Build history of the part. All positions in model axes, mm. A direction names the side the tool comes from. Round coordinates to 2 decimals unless told otherwise and drop trailing zeros. Loops run counter-clockwise (first coordinate to the right, second up) from the corner with the lowest first, then second, coordinate; pieces in that order, holes last. Notation, with made-up numbers: (-27.75, 80) - (7.25, 80) arc R29 cw to (7.25, 119) - close; hole circle Ø9 at (54, 23.25). An arc over 180 degrees is marked (long way). Answer as CSV lines item,"result". Start each with the question number.
```python
from build123d import *

# Parameters (mm, degrees)
F0_W           = 203.2
F0_H           = 76.2
F1_DEPTH       = 50.8
F3_D           = 13.4874
F3_CBORE_D     = 22.225
F3_CBORE_DEPTH = 38.1


with BuildPart() as f1:
    # F0 (on Top) → F1 (new body)
    with BuildSketch(Plane.XY):
        Rectangle(F0_W, F0_H)
    extrude(amount=F1_DEPTH)

    # F3 (through all)
    with Locations(Plane.XY.offset(50.8)):
        with Locations((-49.2125, -14.224), (49.2125, -14.224)):
            CounterBoreHole(F3_D / 2, F3_CBORE_D / 2, F3_CBORE_DEPTH)


solid = f1.part
```
Q1. Wall check: probe 1 along X at (y, z) = (-5, 39); probe 2 along Z at (x, y) = (-40, -10.5); probe 3 along X at (y, z) = (-9.5, 19). Give the ranges that are in metal, low to high. Write a range as [from, to].
Q2. Two-plate mould, pull along X, no slides. Class faces 1 (the cylindrical face through (42.983, -16.807, 6.261)), 2 (the flat face through (-1, 38.1, 25)), 3 (the flat face through (101.6, -1, 25)): released by +X, released by -X, zero draft, split by the parting line, or undercut.
Q3. Band-saw the part on B-B, the plane y = -10. List the corners of the cut face in (x, z), then the cut area to 3 significant figures.
Q4. Tool access for faces 4 (the flat face through (-101.6, -1, 25)), 5 (the cylindrical face through (-50.659, -3.206, 32.017)): list every direction of +Z, -Z, +X, -X, +Y, -Y with a clear straight run to the whole face (end or side of a thin tool).
Q5. Band-saw the part on C-C, the plane z = 39. List the corners of the cut face in (x, y) (1 decimal).
Q6. Band-saw the part on A-A, the plane x = -48. List the corners of the cut face in (y, z).
Q7. Pin check, flat tip, straight feed: pin 1 Ø6.5 at (x, y) = (-53.5, -10.5) entering from +Z. Stop position of the tip, or through.
Reported:
1,probe 1,"x = [-101.6, -55.41], [-43.02, 43.02], [55.41, 101.6]"
1,probe 2,"z = [0, 12.7]"
1,probe 3,"x = [-101.6, -59.27], [-39.15, 39.15], [59.27, 101.6]"
2,face 1,"undercut"
2,face 2,"zero draft"
2,face 3,"released by +X"
3,outline,"(-101.6, 0) - (-54.47, 0) - (-54.47, 12.7) - (-59.49, 12.7) - (-59.49, 50.8) - (-101.6, 50.8) - close; (-43.96, 0) - (43.96, 0) - (43.96, 12.7) - (38.93, 12.7) - (38.93, 50.8) - (-38.93, 50.8) - (-38.93, 12.7) - (-43.96, 12.7) - close; (54.47, 0) - (101.6, 0) - (101.6, 50.8) - (59.49, 50.8) - (59.49, 12.7) - (54.47, 12.7) - close"
3,area,"8,490 mm2"
4,face 4,"+Z, -Z, -X, +Y, -Y"
4,face 5,"+Z"
5,outline,"(-101.6, -38.1) - (101.6, -38.1) - (101.6, 38.1) - (-101.6, 38.1) - close; hole circle Ø22.2 at (-49.2, -14.2); hole circle Ø22.2 at (49.2, -14.2)"
6,outline,"(-38.1, 0) - (-20.86, 0) - (-20.86, 12.7) - (-25.27, 12.7) - (-25.27, 50.8) - (-38.1, 50.8) - close; (-7.59, 0) - (38.1, 0) - (38.1, 50.8) - (-3.18, 50.8) - (-3.18, 12.7) - (-7.59, 12.7) - close"
7,pin 1,"stops at z = 12.7"
